The model under review builds one solid part; all positions refer to its coordinate system, in mm. Face numbers are marked on the shaded views. A direction names the side the tool comes from. Give positions to 0.01 mm unless a question says otherwise; leave off trailing zeros. Write each loop counter-clockwise with the first axis right and the second up, starting at its lowest first coordinate (ties: lowest second). Pieces come first, ordered by that corner, then holes. Notation, with made-up numbers: (-32.5, 64) -> (-12.5, 64) arc R19 cw to (-12.5, 75) -> close; hole circle Ø5 at (64.5, 3.25). An arc over 180 degrees is marked (long way). Use CSV: the item, a comma, the result in double quotes.
```python
from build123d import *
from build123d.topology import SkipClean

# Parameters (mm, degrees)
ESQUISSE2_R                                      = 31.5
ESQUISSE2_W                                      = 32
ESQUISSE2_H                                      = 32
BOSS_EXTRU_1_DEPTH                               = 3
BOSS_EXTRU_2_START                               = -100
ESQUISSE4_R                                      = 35
ESQUISSE4_R_2                                    = 31.5
BOSS_EXTRU_2_DEPTH                               = 100
BOSS_EXTRU_3_OUTLINE_R                           = 31.5
BOSS_EXTRU_3_OUTLINE_W                           = 43
BOSS_EXTRU_3_OUTLINE_H                           = 42.5
BOSS_EXTRU_3_DEPTH                               = 97
ESQUISSE6_R                                      = 31.5
ENL_V_MAT_EXTRU_1_DEPTH                          = 10
ESQUISSE7_R                                      = 49
ESQUISSE7_R_2                                    = 35
BOSS_EXTRU_4_DEPTH                               = 10
BOSS_EXTRU_5_START                               = 30
BOSS_EXTRU_5_DEPTH                               = 30
BOSS_EXTRU_6_START                               = 16
BOSS_EXTRU_6_DEPTH                               = 16
CONG_1_R                                         = 10
ESQUISSE11_W                                     = 137.068824
ESQUISSE11_H                                     = 50.889867
ENL_V_MAT_EXTRU_2_DEPTH                          = 153
CHAMBRAGE_POUR_VIS_T_TE_RONDE_6_PANS_D           = 5.3
CHAMBRAGE_POUR_VIS_T_TE_RONDE_6_PANS_DEPTH       = 18
CHAMBRAGE_POUR_VIS_T_TE_RONDE_6_PANS_CBORE_D     = 10.5
CHAMBRAGE_POUR_VIS_T_TE_RONDE_6_PANS_CBORE_DEPTH = 2.75
CHAMBRAGE_POUR_VIS_T_TE_RONDE_6_PANS_TIP         = 1.592281
ESQUISSE18_R                                     = 2.6
ENL_V_MAT_EXTRU_4_DEPTH                          = 25
ESQUISSE19_R                                     = 4.6
ENL_V_MAT_EXTRU_5_DEPTH                          = 25
ENL_V_START                                      = -90
ENL_V_MAT_EXTRU_6_DEPTH                          = 90


# Read off the part's stored shape, not the designer's step: Boss.-Extru.3
with BuildPart() as part:
    # Esquisse2 → Boss.-Extru.1 (new body)
    with BuildSketch(Plane.XY):
        Circle(ESQUISSE2_R)
        with Locations((0.409228, -1.432297)):
            Rectangle(ESQUISSE2_W, ESQUISSE2_H, mode=Mode.SUBTRACT)
    extrude(amount=BOSS_EXTRU_1_DEPTH)

    # Esquisse4 → Boss.-Extru.2 (add)
    with BuildSketch(Plane.XY.offset(3).offset(BOSS_EXTRU_2_START)):
        Circle(ESQUISSE4_R)
        Circle(ESQUISSE4_R_2, mode=Mode.SUBTRACT)
    extrude(amount=BOSS_EXTRU_2_DEPTH)

    # Boss.-Extru.3 outline → Boss.-Extru.3 (add)
    with BuildSketch(Plane(origin=(0, 0, 0), x_dir=(-1, 0, 0), z_dir=(0, 0, -1))):
        Circle(BOSS_EXTRU_3_OUTLINE_R)
        with Locations((-0.409228, -1.182297)):
            Rectangle(BOSS_EXTRU_3_OUTLINE_W, BOSS_EXTRU_3_OUTLINE_H, mode=Mode.SUBTRACT)
    extrude(amount=BOSS_EXTRU_3_DEPTH)

    # Esquisse6 → Enlèv. mat.-Extru.1 (cut)
    with BuildSketch(Plane(origin=(0, 0, -97), x_dir=(-1, 0, 0), z_dir=(0, 0, -1))):
        Circle(ESQUISSE6_R)
    extrude(amount=-ENL_V_MAT_EXTRU_1_DEPTH, mode=Mode.SUBTRACT)

    # Esquisse7 → Boss.-Extru.4 (add)
    with BuildSketch(Plane(origin=(0, 0, -97), x_dir=(-1, 0, 0), z_dir=(0, 0, -1))):
        Circle(ESQUISSE7_R)
        with Locations(Location((0, 0, 0), (0, 0, 180))):
            Circle(ESQUISSE7_R_2, mode=Mode.SUBTRACT)
    extrude(amount=-BOSS_EXTRU_4_DEPTH)

    # Esquisse8 → Boss.-Extru.5 (add)
    with SkipClean():  # the faces are left unmerged after this step: merging them gives an invalid solid
        with BuildSketch(Plane(origin=(0, 0, -97), x_dir=(-1, 0, 0), z_dir=(0, 0, -1)).offset(BOSS_EXTRU_5_START)):
            with BuildLine():
                Line((-47.96874, 10), (-29.870554, 10))
                ThreePointArc((-29.870554, 10), (-31.5, 0), (-29.870554, -10))
                Line((-29.870554, -10), (-47.96874, -10))
                ThreePointArc((-47.96874, -10), (-49, 0), (-47.96874, 10))
            make_face()
            with BuildLine():
                Line((29.870554, 10), (47.96874, 10))
                ThreePointArc((47.96874, 10), (49, 0), (47.96874, -10))
                Line((47.96874, -10), (29.870554, -10))
                ThreePointArc((29.870554, -10), (31.5, 0), (29.870554, 10))
            make_face()
        extrude(amount=-BOSS_EXTRU_5_DEPTH)

    # Esquisse10 → Boss.-Extru.6 (add)
    with SkipClean():  # the faces are left unmerged after this step: merging them gives an invalid solid
        with BuildSketch(Plane(origin=(0, 0, -127), x_dir=(-1, 0, 0), z_dir=(0, 0, -1)).offset(BOSS_EXTRU_6_START)):
            with BuildLine():
                Line((47.96874, 10), (-47.96874, 10))
                ThreePointArc((-47.96874, 10), (-49, 0), (-47.96874, -10))
                Line((-47.96874, -10), (47.96874, -10))
                ThreePointArc((47.96874, -10), (49, 0), (47.96874, 10))
            make_face()
        extrude(amount=-BOSS_EXTRU_6_DEPTH)

    # Congé1
    cong_1_edges = [part.edges().sort_by_distance(p)[0] for p in [
        (-49, 0, -143),
        (49, 0, -143),
    ]]
    fillet(cong_1_edges, radius=CONG_1_R)

    # Esquisse11 → Enlèv. mat.-Extru.2 (cut)
    with SkipClean():  # the faces are left unmerged after this step: merging them gives an invalid solid
        with BuildSketch(Plane(origin=(0, 0, -143), x_dir=(-1, 0, 0), z_dir=(0, 0, -1))):
            with Locations((0, -25.444933)):
                Rectangle(ESQUISSE11_W, ESQUISSE11_H)
        extrude(amount=-ENL_V_MAT_EXTRU_2_DEPTH, mode=Mode.SUBTRACT)

    # Chambrage pour Vis à tête ronde à 6 pans creux M51
    with Locations(Plane(origin=(0, 10, 0), x_dir=(1, 0, 0), z_dir=(0, 1, 0))):
        with Locations((-38.919647, 112), (38.919647, 112), (0, 135)):
            CounterBoreHole(CHAMBRAGE_POUR_VIS_T_TE_RONDE_6_PANS_D / 2, CHAMBRAGE_POUR_VIS_T_TE_RONDE_6_PANS_CBORE_D / 2, CHAMBRAGE_POUR_VIS_T_TE_RONDE_6_PANS_CBORE_DEPTH, depth=CHAMBRAGE_POUR_VIS_T_TE_RONDE_6_PANS_DEPTH)
            with Locations((0, 0, -(CHAMBRAGE_POUR_VIS_T_TE_RONDE_6_PANS_DEPTH + CHAMBRAGE_POUR_VIS_T_TE_RONDE_6_PANS_TIP / 2))):  # 118° drill point
                Cone(0, CHAMBRAGE_POUR_VIS_T_TE_RONDE_6_PANS_D / 2, CHAMBRAGE_POUR_VIS_T_TE_RONDE_6_PANS_TIP, mode=Mode.SUBTRACT)

    # Esquisse18 → Enlèv. mat.-Extru.4 (cut, symmetric)
    with SkipClean():  # the faces are left unmerged after this step: merging them gives an invalid solid
        with BuildSketch(Plane(origin=(0, 15, 0), x_dir=(-1, 0, 0), z_dir=(0, -1, 0))):
            with Locations(Location((28, 12, 0), (0, 0, 90))):
                Circle(ESQUISSE18_R)
            with Locations(Location((-28, 12, 0), (0, 0, 90))):
                Circle(ESQUISSE18_R)
            with Locations(Location((28, 72, 0), (0, 0, 90))):
                Circle(ESQUISSE18_R)
            with Locations(Location((-28, 72, 0), (0, 0, 90))):
                Circle(ESQUISSE18_R)
        extrude(amount=ENL_V_MAT_EXTRU_4_DEPTH, both=True, mode=Mode.SUBTRACT)

    # Esquisse19 → Enlèv. mat.-Extru.5 (cut)
    with SkipClean():  # the faces are left unmerged after this step: merging them gives an invalid solid
        with BuildSketch(Plane.ZX.offset(35)):
            with Locations((-72, 28)):
                Circle(ESQUISSE19_R)
            with Locations((-12, 28)):
                Circle(ESQUISSE19_R)
            with Locations((-12, -28)):
                Circle(ESQUISSE19_R)
            with Locations((-72, -28)):
                Circle(ESQUISSE19_R)
        extrude(amount=-ENL_V_MAT_EXTRU_5_DEPTH, mode=Mode.SUBTRACT)

    # Esquisse20 → Enlèv. mat.-Extru.6 (cut)
    with SkipClean():  # the faces are left unmerged after this step: merging them gives an invalid solid
        with BuildSketch(Plane.XY.offset(3).offset(ENL_V_START)):
            with BuildLine():
                Line((-35, 0), (-34, 0))
                ThreePointArc((-34, 0), (0, 34), (34, 0))
                Line((34, 0), (35, 0))
                ThreePointArc((35, 0), (0, 35), (-35, 0))
            make_face()
        extrude(amount=ENL_V_MAT_EXTRU_6_DEPTH, mode=Mode.SUBTRACT)


solid = part.part
```
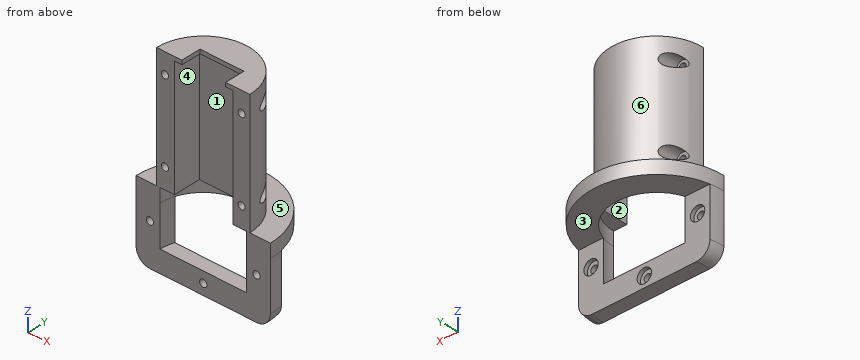
Q1. To check wall thickness, follow probe 1 along Z at (x, y) = (-28, 4); probe 2 along Z at (x, y) = (28, 17); probe 3 along X at (y, z) = (8.65, -112). State the ranges of each line that lie inside material, in increasing order.
Derived:
probe 1,"z = -143 to -127, -87 to -74.6, -69.4 to -14.6, -9.4 to 3"
probe 2,"z = -97 to -76.6, -67.4 to -16.6, -7.4 to 3"
probe 3,"x = -48.23 to -44.17, -33.67 to -30.29, 30.29 to 33.67, 44.17 to 48.23"
Q2. Consider section D-D (z = -27). Write out the cut boundary in (x, y).
Derived:
outline,"(-34, 0) -> (-21.09, 0) -> (-21.09, 20.07) -> (21.91, 20.07) -> (21.91, 0) -> (34, 0) arc R34 ccw to start"
Q3. Machinability: for the marked faces 1, 2 and 3, which of the approach directions +Z, -Z, +X, -X, +Y, -Y give a long, thin tool a straight path to every point of the face, cutting with its end or side? Answer none if there is none.
Derived:
face 1,"-Z, -Y"
face 2,"-Y"
face 3,"-Z, +X, -X, +Y"
Q4. Consider section A-A (x = 0). Write out the cut boundary in (y, z).
Derived:
outline,"(0, -143) -> (10, -143) -> (10, -140.25) -> (7.25, -140.25) -> (7.25, -137.65) -> (0, -137.65) -> close; (0, -132.35) -> (7.25, -132.35) -> (7.25, -129.75) -> (10, -129.75) -> (10, -127) -> (0, -127) -> close; (14.57, 0) -> (20.07, 0) -> (20.07, -87) -> (31.5, -87) -> (31.5, -97) -> (49, -97) -> (49, -87) -> (34, -87) -> (34, 3) -> (14.57, 3) -> close"
Q5. Consider section B-B (z = -100.5). Write out the cut boundary in (x, y).
Derived:
outline,"(-49, 0) -> (-31.5, 0) arc R31.5 cw to (-29.87, 10) -> (-47.97, 10) arc R49 ccw to start; (29.87, 10) arc R31.5 cw to (31.5, 0) -> (49, 0) arc R49 ccw to (47.97, 10) -> close"
Q6. Insertion check: pin 1 (3 mm diameter, centred on x = -37, z = -114, fed in from +Y); pin 2 (2 mm diameter, centred on y = 31.5, z = -63, fed in from +X) (3 decimals); pin 3 (1.5 mm diameter, centred on x = -35.5, y = 7, fed in from +Z). Each pin has a flat end and moves straight along its axis. Give the tip position at first contact, or say it passes through.
Derived:
pin 1,"stops at y = 7.25"
pin 2,"stops at x = 15.025"
pin 3,"stops at z = -87"
Q7. The part is to be moulded in two halves that separate along X. For the marked faces 4, 5 and 6, say which applies: pulls with the +X half, pulls with the -X half, needs draft (parallel to the pull), parting line crosses it, or undercut.
Derived:
face 4,"undercut"
face 5,"needs draft"
face 6,"parting line crosses it"
Q8. Consider section C-C (x = 28). Write out the cut boundary in (y, z), then the cut area to 3 significant figures.
Derived:
outline,"(0, -143) -> (10, -143) -> (10, -127) -> (0, -127) -> close; (0, -87) -> (14.43, -87) -> (14.43, -97) -> (40.21, -97) -> (40.21, -87) -> (19.29, -87) -> (19.29, -76.6) -> (10, -76.6) -> (10, -74.6) -> (0, -74.6) -> close; (0, -69.4) -> (10, -69.4) -> (10, -67.4) -> (19.29, -67.4) -> (19.29, -16.6) -> (10, -16.6) -> (10, -14.6) -> (0, -14.6) -> close; (0, -9.4) -> (10, -9.4) -> (10, -7.4) -> (19.29, -7.4) -> (19.29, 3) -> (0, 3) -> close"
area,"1,880 mm2"
